Geometry: final body of the model. Coordinates: model frame, mm. A direction names the side the tool comes from. Give positions to 0.01 mm unless a question says otherwise; leave off trailing zeros. Write each loop counter-clockwise with the first axis right and the second up, starting at its lowest first coordinate (ties: lowest second). Pieces come first, ordered by that corner, then holes. Notation, with made-up numbers: M 58.5,36.25 L 99.5,36.25 A23 ccw 99.5,44.25 Z; hole C 13,22.25 d6. An arc over 180 degrees is marked long. Use a Markdown table: item, result. Add a question column.
(1) Draft query along X for faces 1 (the flat face through (6, 0, 0)), 2 (the cylindrical face through (-5.1, 6.93, 1.52)), 3 (the cylindrical face through (32.18, -0.37, 1.52)). Return one class per face: released by +X, released by -X, zero draft, split by the parting line, or undercut.
(2) Reachability of faces 4 (the flat face through (34, 6, -4)), 5 (the flat face through (12.75, 3, 1)), 6 (the flat face through (40, 0, 1)) from +Z, -Z, +X, -X, +Y, -Y: full face, straight path, thin tool, end or side. Return the list, or none.
(3) Cut plane A-A (z = -9). Output: boundary loops of the cut face in (x, y), plus the area to 3 significant figures.
(4) Cut plane B-B (x = -15.5). Output: boundary loops of the cut face in (y, z), plus the area to 4 significant figures.
(5) Pin query (flat end, axial travel): pin 1 Ø0.9 at (x, z) = (38.5, 1) entering from -Y; pin 2 Ø1.5 at (y, z) = (6.5, -2.5) entering from -X; pin 3 Ø3 at (x, z) = (42.5, -9) entering from +Y; pin 4 Ø5 at (x, z) = (45, -10) entering from -Y. Return the tip coordinate at first contact, or that it passes through.
(6) Cut plane C-C (z = -3.5). Output: boundary loops of the cut face in (x, y), plus the area to 3 significant figures.
(7) Material intervals for L1, parallel to Z at x = 42.5, y = 5.2; L2, parallel to X at y = -2.5, z = 1.5; L3, parallel to Z at x = -11, y = 0.5, sorted ascending.
```python
from build123d import *

# Parameters (mm, degrees)
PAD_DEPTH    = 3
SKETCH001_W  = 17
SKETCH001_H  = 3
PAD001_DEPTH = 16
SKETCH002_R  = 2.6
POCKET_DEPTH = 3.001
FILLET_R     = 8
FILLET002_R  = 7
FILLET003_R  = 4
FILLET004_R  = 5
FILLET005_R  = 2


with BuildPart() as part:
    # Sketch → Pad (new body)
    with BuildSketch(Plane.XY):
        with BuildLine():
            ThreePointArc((-4.5, 0), (0, -4.5), (4.5, 0))
            Line((4.5, 0), (4.5, 7.5))
            Line((4.5, 7.5), (12.75, 7.5))
            Line((12.75, 0), (12.75, 7.5))
            ThreePointArc((12.75, 0), (15.5, -2.75), (18.25, 0))
            Line((18.25, 0), (18.25, 7.5))
            Line((18.25, 7.5), (51, 7.5))
            Line((51, 0), (51, 7.5))
            Line((32, 0), (51, 0))
            Line((23.5, -8.5), (32, 0))
            Line((-23.5, -8.5), (23.5, -8.5))
            Line((-23.5, 7.5), (-23.5, -8.5))
            Line((-23.5, 7.5), (-18.25, 7.5))
            Line((-18.25, 0), (-18.25, 7.5))
            ThreePointArc((-18.25, 0), (-15.5, -2.75), (-12.75, 0))
            Line((-12.75, 0), (-12.75, 7.5))
            Line((-12.75, 7.5), (-4.5, 7.5))
            Line((-4.5, 0), (-4.5, 7.5))
        make_face()
    extrude(amount=PAD_DEPTH)

    # Sketch001 (on Face19 of Pad) → Pad001 (join)
    with BuildSketch(Plane(origin=(0, 0, 0), x_dir=(1, 0, 0), z_dir=(0, 0, -1))):
        with Locations((42.5, -6)):
            Rectangle(SKETCH001_W, SKETCH001_H)
    extrude(amount=PAD001_DEPTH)

    # Sketch002 (on Face13 of Pad001) → Pocket (cut, through all)
    with BuildSketch(Plane.XZ.offset(-4.5)):
        with Locations((42.5, -9)):
            Circle(SKETCH002_R)
    extrude(amount=-POCKET_DEPTH, mode=Mode.SUBTRACT)

    # Fillet
    fillet_edges = [part.edges().sort_by_distance(p)[0] for p in [
        (34, 6, -16),
        (51, 6, -16),
    ]]
    fillet(fillet_edges, radius=FILLET_R)

    # Fillet002
    fillet002_edges = [part.edges().sort_by_distance(p)[0] for p in [
        (-23.5, -8.5, 1.5),
    ]]
    fillet(fillet002_edges, radius=FILLET002_R)

    # Fillet003
    fillet003_edges = [part.edges().sort_by_distance(p)[0] for p in [
        (51, 0, 1.5),
    ]]
    fillet(fillet003_edges, radius=FILLET003_R)

    # Fillet004
    fillet004_edges = [part.edges().sort_by_distance(p)[0] for p in [
        (23.5, -8.5, 1.5),
        (32, 0, 1.5),
    ]]
    fillet(fillet004_edges, radius=FILLET004_R)

    # Fillet005
    fillet005_edges = [part.edges().sort_by_distance(p)[0] for p in [
        (-23.5, 7.5, 1.5),
        (-18.25, 7.5, 1.5),
        (-12.75, 7.5, 1.5),
        (-4.5, 7.5, 1.5),
        (4.5, 7.5, 1.5),
        (12.75, 7.5, 1.5),
        (18.25, 7.5, 1.5),
    ]]
    fillet(fillet005_edges, radius=FILLET005_R)


solid = part.part
```
Answer list:
| question | item | result |
|---|---|---|
| 1 | face 1 | zero draft |
| 1 | face 2 | undercut |
| 1 | face 3 | released by +X |
| 2 | face 4 | -Z, -X, +Y, -Y |
| 2 | face 5 | +Z, -Z, +Y |
| 2 | face 6 | +Z, -Z, +X, -Y |
| 3 | outline | M 34.06,4.5 L 39.9,4.5 L 39.9,7.5 L 34.06,7.5 Z; M 45.1,4.5 L 50.94,4.5 L 50.94,7.5 L 45.1,7.5 Z |
| 3 | area | 35.0 mm² |
| 4 | outline | M -8.5,0 L -2.75,0 L -2.75,3 L -8.5,3 Z |
| 4 | area | 17.25 mm² |
| 5 | pin 1 | y = 0 |
| 5 | pin 2 | x = 34 |
| 5 | pin 3 | through |
| 5 | pin 4 | y = 4.5 |
| 6 | outline | M 34,4.5 L 51,4.5 L 51,7.5 L 34,7.5 Z |
| 6 | area | 51.0 mm² |
| 7 | L1 | -16 to -11.6, -6.4 to 3 |
| 7 | L2 | -23.43 to -16.65, -14.35 to -3.74, 3.74 to 14.35, 16.65 to 29.5 |
| 7 | L3 | 0 to 3 |
